Check sheet for the modelled part. Datum: model origin and axes. Units: mm. A direction names the side the tool comes from. Round coordinates to 2 decimals unless told otherwise and drop trailing zeros. Write each loop counter-clockwise with the first axis right and the second up, starting at its lowest first coordinate (ties: lowest second). Pieces come first, ordered by that corner, then holes. Notation, with made-up numbers: (46, 87) -> (95, 87) arc R26 cw to (95, 117) -> close; hole circle Ø4 at (-23.75, 52.5). An arc over 180 degrees is marked (long way). Answer as a JSON object with one key per item and string values. Group by question number.
```python
from build123d import *

# Parameters (mm, degrees)
SKETCH1_R               = 0.915
BOSS_EXTRUDE1_DEPTH     = 4.37
BOSS_EXTRUDE1_2_DEPTH   = 4.37
BOSS_EXTRUDE1_3_DEPTH   = 4.37
BOSS_EXTRUDE1_4_DEPTH   = 4.37
BOSS_EXTRUDE2_START     = 4.37
SKETCH1_3_R             = 4.7
SKETCH1_3_R_2           = 0.915
BOSS_EXTRUDE2_DEPTH     = 15
CUT_EXTRUDE1_DEPTH      = 245.162747978
SKETCH1_6_R             = 2.625
SKETCH1_6_R_2           = 0.75
CUT_EXTRUDE4_DEPTH      = 245.162747978
SKETCH5_R               = 1.6
BOSS_EXTRUDE4_DEPTH     = 2
LPATTERN1_COUNT         = 2
LPATTERN1_PITCH         = 73
LPATTERN1_COL_COUNT     = 2
LPATTERN1_COL_PITCH     = 73
MIRROR1_COPY_1_SKETCH_R = 1.6
MIRROR1_COPY_1_DEPTH    = 2
MIRROR1_COPY_2_SKETCH_R = 1.6
MIRROR1_COPY_2_DEPTH    = 2


with BuildPart() as part:
    # Sketch1 → Boss-Extrude1 (new body)
    with BuildSketch(Plane(origin=(0, 0, 0), x_dir=(1, 0, 0), z_dir=(0, 1, 0))):
        with Locations(Location((-1.117435623, 2.697728235, 0), (0, 0, 270))):
            Circle(SKETCH1_R)
    extrude(amount=BOSS_EXTRUDE1_DEPTH)



with BuildPart() as body_2:
    # Sketch1 → Boss-Extrude1 2 (new body)
    with BuildSketch(Plane(origin=(0, 0, 0), x_dir=(1, 0, 0), z_dir=(0, 1, 0))):
        with Locations(Location((-1.117435623, -2.697728235, 0), (0, 0, 270))):
            Circle(SKETCH1_R)
    extrude(amount=BOSS_EXTRUDE1_2_DEPTH)


with BuildPart() as body_3:
    # Sketch1 → Boss-Extrude1 3 (new body)
    with BuildSketch(Plane(origin=(0, 0, 0), x_dir=(1, 0, 0), z_dir=(0, 1, 0))):
        with Locations(Location((1.117435623, 2.697728235, 0), (0, 0, 270))):
            Circle(SKETCH1_R)
    extrude(amount=BOSS_EXTRUDE1_3_DEPTH)


with BuildPart() as body_4:
    # Sketch1 → Boss-Extrude1 4 (new body)
    with BuildSketch(Plane(origin=(0, 0, 0), x_dir=(1, 0, 0), z_dir=(0, 1, 0))):
        with Locations(Location((1.117435623, -2.697728235, 0), (0, 0, 270))):
            Circle(SKETCH1_R)
    extrude(amount=BOSS_EXTRUDE1_4_DEPTH)


with BuildPart() as part_1:
    add(part.part)

    add(body_2.part)  # Boss-Extrude2 merges body 2

    add(body_3.part)  # Boss-Extrude2 merges body 3

    add(body_4.part)  # Boss-Extrude2 merges body 4
    # Sketch1<3> → Boss-Extrude2 (add)
    # profile 1 of 5: a face of its own
    with BuildSketch(Plane(origin=(0, 0, 0), x_dir=(1, 0, 0), z_dir=(0, 1, 0)).offset(BOSS_EXTRUDE2_START)):
        with Locations(Location((0, 0, 0), (0, 0, 270))):
            Circle(SKETCH1_3_R)
        with Locations(Location((-1.117435623, -2.697728235, 0), (0, 0, 270))):
            Circle(SKETCH1_3_R_2, mode=Mode.SUBTRACT)
        with Locations(Location((1.117435623, -2.697728235, 0), (0, 0, 270))):
            Circle(SKETCH1_3_R_2, mode=Mode.SUBTRACT)
        with Locations(Location((1.117435623, 2.697728235, 0), (0, 0, 270))):
            Circle(SKETCH1_3_R_2, mode=Mode.SUBTRACT)
        with Locations(Location((-1.117435623, 2.697728235, 0), (0, 0, 270))):
            Circle(SKETCH1_3_R_2, mode=Mode.SUBTRACT)
    # profile 2 of 5: a face of its own
    with BuildSketch(Plane(origin=(0, 0, 0), x_dir=(1, 0, 0), z_dir=(0, 1, 0)).offset(BOSS_EXTRUDE2_START)):
        with Locations(Location((-1.117435623, -2.697728235, 0), (0, 0, 270))):
            Circle(SKETCH1_3_R_2)
    # profile 3 of 5: a face of its own
    with BuildSketch(Plane(origin=(0, 0, 0), x_dir=(1, 0, 0), z_dir=(0, 1, 0)).offset(BOSS_EXTRUDE2_START)):
        with Locations(Location((1.117435623, -2.697728235, 0), (0, 0, 270))):
            Circle(SKETCH1_3_R_2)
    # profile 4 of 5: a face of its own
    with BuildSketch(Plane(origin=(0, 0, 0), x_dir=(1, 0, 0), z_dir=(0, 1, 0)).offset(BOSS_EXTRUDE2_START)):
        with Locations(Location((1.117435623, 2.697728235, 0), (0, 0, 270))):
            Circle(SKETCH1_3_R_2)
    # profile 5 of 5: a face of its own
    with BuildSketch(Plane(origin=(0, 0, 0), x_dir=(1, 0, 0), z_dir=(0, 1, 0)).offset(BOSS_EXTRUDE2_START)):
        with Locations(Location((-1.117435623, 2.697728235, 0), (0, 0, 270))):
            Circle(SKETCH1_3_R_2)
    extrude(amount=BOSS_EXTRUDE2_DEPTH)


with BuildPart() as body_2_2:
    # Sweep1: sweep along a path in Sketch4
    with BuildLine(Plane(origin=(0, 0, 0), x_dir=(1, 0, 0), z_dir=(0, 1, 0))) as sweep1_path:
        Line((-96, -197.7), (96, -197.7))
        Line((96, -197.7), (96, -5.7))
        Line((96, -5.7), (-96, -5.7))
        Line((-96, -5.7), (-96, -197.7))
    # Sketch2 → Sweep1 (sweep)
    with BuildSketch(Plane(origin=(0, 0, 0), x_dir=(0, 0, -1), z_dir=(1, 0, 0))):
        Polygon((-5.7, -4), (-5.7, 13.85), (12.15, -4), align=None)
    sweep(path=sweep1_path.line, transition=Transition.RIGHT)

    # Combine2: cut part
    add(part_1.part, mode=Mode.SUBTRACT)

    # Sketch3 → Cut-Extrude1 (cut, through all)
    with BuildSketch(Plane(origin=(0, 0, 0), x_dir=(1, 0, 0), z_dir=(0, 1, 0))):
        Polygon((-15.05, -5.7), (15.05, -5.7), (4.35, 5), (-4.35, 5), align=None)
    extrude(amount=-CUT_EXTRUDE1_DEPTH, mode=Mode.SUBTRACT)

    # Sketch1<6> → Cut-Extrude4 (cut, through all)
    # profile 1 of 4: a face of its own
    with BuildSketch(Plane(origin=(0, 0, 0), x_dir=(1, 0, 0), z_dir=(0, 1, 0))):
        with Locations(Location((-7.4, -2.3, 0), (0, 0, 90))):
            Circle(SKETCH1_6_R)
    # profile 2 of 4: a face of its own
    with BuildSketch(Plane(origin=(0, 0, 0), x_dir=(1, 0, 0), z_dir=(0, 1, 0))):
        with Locations(Location((7.4, -2.3, 0), (0, 0, 90))):
            Circle(SKETCH1_6_R)
        with Locations((8.9, -2.3)):
            Circle(SKETCH1_6_R_2, mode=Mode.SUBTRACT)
        with Locations((5.9, -2.3)):
            Circle(SKETCH1_6_R_2, mode=Mode.SUBTRACT)
    # profile 3 of 4: a face of its own
    with BuildSketch(Plane(origin=(0, 0, 0), x_dir=(1, 0, 0), z_dir=(0, 1, 0))):
        with Locations((5.9, -2.3)):
            Circle(SKETCH1_6_R_2)
    # profile 4 of 4: a face of its own
    with BuildSketch(Plane(origin=(0, 0, 0), x_dir=(1, 0, 0), z_dir=(0, 1, 0))):
        with Locations((8.9, -2.3)):
            Circle(SKETCH1_6_R_2)
    extrude(amount=CUT_EXTRUDE4_DEPTH, mode=Mode.SUBTRACT)

    # Sketch5 → Boss-Extrude4 (add)
    with BuildSketch(Plane(origin=(0, 0, 0), x_dir=(1, 0, 0), z_dir=(0, 1, 0))):
        with BuildLine():
            ThreePointArc((-84, -106.3), (-79.4, -101.7), (-84, -97.1))
            Line((-84, -97.1), (-92, -97.1))
            ThreePointArc((-92, -97.1), (-94.828427125, -95.928427125), (-96, -93.1))
            Line((-96, -93.1), (-96, -110.3))
            ThreePointArc((-96, -110.3), (-94.828427125, -107.471572875), (-92, -106.3))
            Line((-92, -106.3), (-84, -106.3))
        make_face()
        with Locations(Location((-84, -101.7, 0), (0, 0, 270))):
            Circle(SKETCH5_R, mode=Mode.SUBTRACT)
    boss_extrude4 = extrude(amount=-BOSS_EXTRUDE4_DEPTH)

    # LPattern1: Boss-Extrude4 ×2
    with Locations(*[(0, 0, -i * LPATTERN1_PITCH) for i in range(1, LPATTERN1_COUNT)]):
        add(boss_extrude4)

    # LPattern1 col: Boss-Extrude4 ×2
    with Locations(*[(0, 0, i * LPATTERN1_COL_PITCH) for i in range(1, LPATTERN1_COL_COUNT)]):
        add(boss_extrude4)

    # Mirror1: Boss-Extrude4 across plane
    add(boss_extrude4.mirror(Plane(origin=(0, 0, 0), x_dir=(0, 0, 1), z_dir=(1, 0, 0))))

    # Mirror1 copy 1 sketch → Mirror1 copy 1 (add)
    with BuildSketch(Plane(origin=(0, 0, -73), x_dir=(-1, 0, 0), z_dir=(0, 1, 0))):
        with BuildLine():
            ThreePointArc((-84, 106.3), (-79.4, 101.7), (-84, 97.1))
            Line((-84, 97.1), (-92, 97.1))
            ThreePointArc((-92, 97.1), (-94.828427125, 95.928427125), (-96, 93.1))
            Line((-96, 93.1), (-96, 110.3))
            ThreePointArc((-96, 110.3), (-94.828427125, 107.471572875), (-92, 106.3))
            Line((-92, 106.3), (-84, 106.3))
        make_face()
        with Locations((-84, 101.7)):
            Circle(MIRROR1_COPY_1_SKETCH_R, mode=Mode.SUBTRACT)
    extrude(amount=-MIRROR1_COPY_1_DEPTH)

    # Mirror1 copy 2 sketch → Mirror1 copy 2 (add)
    with BuildSketch(Plane(origin=(0, 0, 73), x_dir=(-1, 0, 0), z_dir=(0, 1, 0))):
        with BuildLine():
            ThreePointArc((-84, 106.3), (-79.4, 101.7), (-84, 97.1))
            Line((-84, 97.1), (-92, 97.1))
            ThreePointArc((-92, 97.1), (-94.828427125, 95.928427125), (-96, 93.1))
            Line((-96, 93.1), (-96, 110.3))
            ThreePointArc((-96, 110.3), (-94.828427125, 107.471572875), (-92, 106.3))
            Line((-92, 106.3), (-84, 106.3))
        make_face()
        with Locations((-84, 101.7)):
            Circle(MIRROR1_COPY_2_SKETCH_R, mode=Mode.SUBTRACT)
    extrude(amount=-MIRROR1_COPY_2_DEPTH)


solid = body_2_2.part
```
(1) Section check A-A on x = -27. Record the cut outline in (y, z), then the cut area to 3 significant figures.
(2) Access from +Z, -Z, +X, -X, +Y, -Y to the whole of each face (thin tool, end or side, straight path). Record for faces 5 (the flat face through (105.05, 4.8, 100.11)), 6 (the flat face through (-105.05, 4.8, 103.29)), 7 (the flat face through (1, 5, 197.7)), 8 (the flat face through (88, 0, 102)), 9 (the flat face through (-88, -2, 29)).
(3) Section check C-C on x = 7.4. Record the cut outline in (y, z) (3 decimals).
(4) Section check B-B on z = 143. Record the cut outline in (x, y), then the cut area to 3 significant figures.
(5) Go/stop test with flat-tipped pins: pin 1 Ø0.6 at (x, y) = (-89.5, -1) entering from +Z; pin 2 Ø2 at (x, z) = (1.12, 2.7) entering from -Y; pin 3 Ø2 at (x, y) = (86.5, -1) entering from +Z. Record where each tip stops, or that it passes through.
(6) Release check for a two-part mould opening along Z. For faces 1 (the flat face through (-88, 0, 175)), 2 (the flat face through (2, -4, 201)), 3 (the flat face through (-1.59, 2.82, -5.33)), 4 (the flat face through (-1, 5, 5.7)) record: pulls with the +Z half, pulls with the -Z half, needs draft (parallel to the pull), parting line crosses it, or undercut.
(7) Scan lines: line 1 along X through (y, z) = (-0.35, 174.7); line 2 along Z through (x, y) = (-3.5, 12.75); line 3 along Z through (x, y) = (-48.5, 3). Record each from-to range of solid material in increasing order.
Data:
{
 "1": {"outline": "(-4, -12.15) -> (13.85, 5.7) -> (-4, 5.7) -> close; (-4, 197.7) -> (13.85, 197.7) -> (-4, 215.55) -> close", "area": "319 mm²"},
 "2": {"face 5": "+Z, -Z, +X, +Y", "face 6": "+Z, -Z, -X, +Y", "face 7": "+Y, -Y", "face 8": "+Y", "face 9": "-Y"},
 "3": {"outline": "(-4, -12.15) -> (7.825, -0.325) -> (0, -0.325) -> (0, -1.95) -> (-4, -1.95) -> close; (-4, 197.7) -> (13.85, 197.7) -> (-4, 215.55) -> close; (0, 4.925) -> (13.075, 4.925) -> (13.85, 5.7) -> (0, 5.7) -> close"},
 "4": {"outline": "(-113.85, -4) -> (-96, -4) -> (-96, 13.85) -> close; (96, -4) -> (113.85, -4) -> (96, 13.85) -> close", "area": "319 mm²"},
 "5": {"pin 1": "stops at z = 212.85", "pin 2": "stops at y = 0", "pin 3": "stops at z = 213.55"},
 "6": {"face 1": "undercut", "face 2": "needs draft", "face 3": "pulls with the -Z half", "face 4": "undercut"},
 "7": {"line 1": "x = -110.2 to -85.6, -82.4 to -79.4, 79.4 to 82.4, 85.6 to 110.2", "line 2": "z = 4.6 to 5.7, 197.7 to 198.8", "line 3": "z = -5.15 to 5.7, 197.7 to 208.55"}
}
